Answer from the drawing. Dimensions are ordinates in mm from the lowest x, y and z of the part. A direction names the side the tool comes from. Coordinates: 2 decimals unless noted, no trailing zeros. Write each loop counter-clockwise with the first axis right and the second up, starting at its lowest first coordinate (ties: lowest second). Pieces come first, ordered by that corner, then holes. Notation, with made-up numbers: (88.5, 82) -> (110.5, 82) arc R7 cw to (110.5, 90) -> close; hole circle Ø6 at (30, -0.75). An arc over 180 degrees is marked (long way). One line per item, written item: value. Start each with the question number.
1. Find section D-D, the plane z = 98. Write down the section's boundary in (x, y).
2. Find section B-B, the plane z = 25.5. Write down the section's boundary in (x, y).
3. Given P1, Ø12, axis at x = 388.5, y = 136.5, coming from the +Z side, flat-ended and moving along its own axis, determine where the tip first touches the part or whether it passes through.
4. For the marked faces 1 and 2, determine the directions among +Z, -Z, +X, -X, +Y, -Y from which every point of the face is accessible in a straight line to the end or side of a thin tool.
5. Find section C-C, the plane y = 227. Write down the section's boundary in (x, z), and give its area (3 significant figures).
6. Consider line 1 along Y through (x, z) = (175.5, 63); line 2 along Z through (x, y) = (311.5, 67). Determine where each line is inside the solid, lowest interval first.
7. Find section A-A, the plane x = 296.5. Write down the section's boundary in (y, z).
8. For a pull along Y with two mould halves and no side action, classify the marked faces 3, 4 and 5 as pulls with the +Y half, pulls with the -Y half, needs draft (parallel to the pull), parting line crosses it, or undercut.
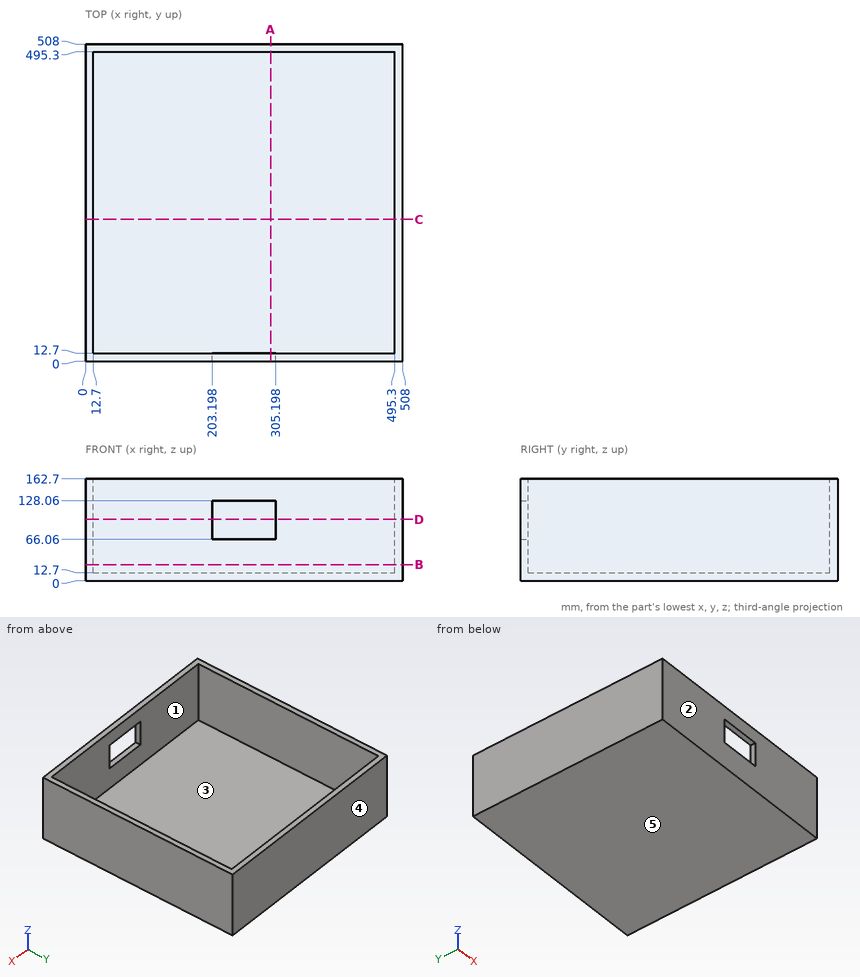
Answer block:
1. outline: (0, 0) -> (203.2, 0) -> (203.2, 12.7) -> (12.7, 12.7) -> (12.7, 495.3) -> (495.3, 495.3) -> (495.3, 12.7) -> (305.2, 12.7) -> (305.2, 0) -> (508, 0) -> (508, 508) -> (0, 508) -> close
2. outline: (0, 0) -> (508, 0) -> (508, 508) -> (0, 508) -> close; hole (12.7, 12.7) -> (495.3, 12.7) -> (495.3, 495.3) -> (12.7, 495.3) -> close
3. P1: stops at z = 12.7
4. face 1: +Z
4. face 2: +Z, -Z, +X, -X, -Y
5. outline: (0, 0) -> (508, 0) -> (508, 162.7) -> (495.3, 162.7) -> (495.3, 12.7) -> (12.7, 12.7) -> (12.7, 162.7) -> (0, 162.7) -> close
5. area: 10,300 mm2
6. line 1: y = 0 to 12.7, 495.3 to 508
6. line 2: z = 0 to 12.7
7. outline: (0, 0) -> (508, 0) -> (508, 162.7) -> (495.3, 162.7) -> (495.3, 12.7) -> (12.7, 12.7) -> (12.7, 66.06) -> (0, 66.06) -> close; (0, 128.06) -> (12.7, 128.06) -> (12.7, 162.7) -> (0, 162.7) -> close
8. face 3: undercut
8. face 4: pulls with the +Y half
8. face 5: needs draft
